Design review of the part built by this model. Coordinates are the model's own, in mm. A direction names the side the tool comes from. Round coordinates to 2 decimals unless told otherwise and drop trailing zeros. Order: outer loops, then holes, each group sorted by start corner. A loop starts at its lowest first (then second) coordinate and runs counter-clockwise, first axis right, second up. Notation, with made-up numbers: (-16, 67.5) - (28, 67.5) arc R16 cw to (28, 93.5) - close; hole circle Ø9 at (17, 16). An arc over 180 degrees is marked (long way). Use CSV: the item, a comma, the result in double quotes.
from build123d import *

# Parameters (mm, degrees)
F0_R     = 52.143145
F1_DEPTH = 254
F2_R     = 33.525148
F3_DEPTH = 254.001
F4_W     = 218.61928
F4_H     = 180.868745
F5_DEPTH = 25.4


with BuildPart() as f1:
    # F0 (on Top) → F1 (new body)
    with BuildSketch(Plane.XY):
        with Locations((5.621463, -5.621463)):
            Circle(F0_R)
    extrude(amount=F1_DEPTH)

    # F2 (on face) → F3 (cut, through all)
    with BuildSketch(Plane.XY.offset(254)):
        with Locations((5.621463, -5.621463)):
            Circle(F2_R)
    extrude(amount=-F3_DEPTH, mode=Mode.SUBTRACT)

    # F4 (on Top) → F5 (join)
    with BuildSketch(Plane.XY):
        with Locations((15.006397, -13.178111)):
            Rectangle(F4_W, F4_H)
    extrude(amount=F5_DEPTH)


solid = f1.part
1) Insertion check: pin 1 Ø3 at (x, z) = (21.5, 31.5) entering from -Y; pin 2 Ø12 at (x, z) = (12.5, 70.5) entering from +Y; pin 3 Ø12 at (x, z) = (40, 184) entering from +Y. Each pin has a flat end and moves straight along its axis. Give the tip position at first contact, or say it passes through.
Data:
pin 1,"stops at y = -55.74"
pin 2,"stops at y = 46.51"
pin 3,"stops at y = 38.12"
2) To check wall thickness, follow L1, parallel to X at y = -6, z = 157; L2, parallel to Z at x = -85, y = 1.5; L3, parallel to Y at x = -7, z = 222.5. State the ranges of each line that lie inside material, in increasing order. Write a range as from..to.
Data:
L1,"x = -46.52..-27.9, 39.14..57.76"
L2,"z = 0..25.4"
L3,"y = -56.21..-36.68, 25.44..44.97"
3) We need section B-B (x = 101.5). Give the boundary of the cut face in (y, z), then the cut area to 3 significant figures.
Data:
outline,"(-103.61, 0) - (77.26, 0) - (77.26, 25.4) - (-103.61, 25.4) - close"
area,"4,590 mm2"
4) We need section D-D (y = -30). Give the boundary of the cut face in (x, z) (3 decimals), then the cut area to 3 significant figures.
Data:
outline,"(-94.303, 0) - (124.316, 0) - (124.316, 25.4) - (51.715, 25.4) - (51.715, 254) - (28.635, 254) - (28.635, 25.4) - (-17.392, 25.4) - (-17.392, 254) - (-40.472, 254) - (-40.472, 25.4) - (-94.303, 25.4) - close"
area,"16,100 mm2"
5) For faces 1 (the face through (37.6, 4.45, 141.3)), 2 (the face through (13, -12, 0)), list the 3-axis set-ups (+Z, -Z, +X, -X, +Y, -Y) from which the entire face can be reached by the end or side of a thin tool; tool diameter is ignored.
Data:
face 1,"+Z"
face 2,"-Z, +X, -X, +Y, -Y"
6) We need section C-C (z = 96.5). Give the boundary of the cut face in (x, y).
Data:
outline,"circle Ø104.29 at (5.62, -5.62); hole circle Ø67.05 at (5.62, -5.62)"
7) We need section A-A (y = 37). Give the boundary of the cut face in (x, z), then the cut area to 3 significant figures.
Data:
outline,"(-94.3, 0) - (124.32, 0) - (124.32, 25.4) - (35.66, 25.4) - (35.66, 254) - (-24.42, 254) - (-24.42, 25.4) - (-94.3, 25.4) - close"
area,"19,300 mm2"
